```python
from build123d import *

# Parameters (mm, degrees)
BOSS_EXTRUDE1_DEPTH      = 1.5875
BOSS_EXTRUDE1_DEPTH_BACK = 1.5875
FILLET1_R                = 1.524
BOSS_EXTRUDE2_DEPTH      = 0.89581
BOSS_EXTRUDE2_DEPTH_BACK = 0.89581
FILLET2_R                = 1.016


with BuildPart() as part:
    # Sketch1 → Boss-Extrude1 (new, two sides: drawn at the far end of the back side and taken through both)
    with BuildSketch(Plane(origin=(0, 0, 0), x_dir=(1, 0, 0), z_dir=(0, 1, 0)).offset(-BOSS_EXTRUDE1_DEPTH_BACK)):
        with BuildLine():
            Line((-0.068296764, 6.214618695), (-0.068296764, 13.71487153))
            Line((-0.068296764, 13.71487153), (-0.895808533, 13.71487153))
            add(Edge.make_bspline(
                [(-0.895808533, 13.71487153), (-0.895808533, 4.54222596), (-1.588668774, 2.219313027), (-2.088196173, 1.337696034), (0, 0.766240154)],
                knots=[0, 0, 0, 0, 0, 1, 1, 1, 1, 1], degree=4))
            add(Edge.make_bspline(
                [(0.895808533, 13.71487153), (0.895808533, 4.54222596), (1.588668774, 2.219313027), (2.088196173, 1.337696034), (0, 0.766240154)],
                knots=[0, 0, 0, 0, 0, 1, 1, 1, 1, 1], degree=4))
            Line((0.895808533, 13.71487153), (0.068296764, 13.71487153))
            Line((0.068296764, 13.71487153), (0.068296764, 6.214618695))
            add(Edge.make_bspline(
                [(0.690807422, 2.606475487), (0.218071276, 3.482132924), (0.068296764, 6.214618695)],
                knots=[0, 0, 0, 1, 1, 1], degree=2))
            ThreePointArc((0.690807422, 2.606475487), (0, 1.52287153), (-0.690807422, 2.606475487))
            add(Edge.make_bspline(
                [(-0.690807422, 2.606475487), (-0.217222133, 3.738734236), (-0.068296764, 6.214618695)],
                knots=[0, 0, 0, 1, 1, 1], degree=2))
        make_face()
    extrude(amount=BOSS_EXTRUDE1_DEPTH + BOSS_EXTRUDE1_DEPTH_BACK)

    # Fillet1
    fillet1_edges = [part.edges().sort_by_distance(p)[0] for p in [
        (0, -0.79375, -0.766240154),
    ]]
    fillet(fillet1_edges, radius=FILLET1_R)

    # Sketch2 → Boss-Extrude2 (add, two sides: drawn at the far end of the back side and taken through both)
    with BuildSketch(Plane(origin=(0, 0, 0), x_dir=(0, 0, -1), z_dir=(1, 0, 0)).offset(-BOSS_EXTRUDE2_DEPTH_BACK)):
        Polygon((13.71487153, 1.5875), (13.71487153, -1.5875), (13.71487153, -23.8125), (14.73087153, -23.8125), (14.73087153, 1.5875), align=None)
    extrude(amount=BOSS_EXTRUDE2_DEPTH + BOSS_EXTRUDE2_DEPTH_BACK)

    # Fillet2
    fillet2_edges = [part.edges().sort_by_distance(p)[0] for p in [
        (0, 1.5875, -14.73087153),
        (0.482052648, -1.5875, -13.71487153),
        (-0.482052648, -1.5875, -13.71487153),
    ]]
    fillet(fillet2_edges, radius=FILLET2_R - 0.0001)  # a hair under: the kernel refuses the full size


solid = part.part
```
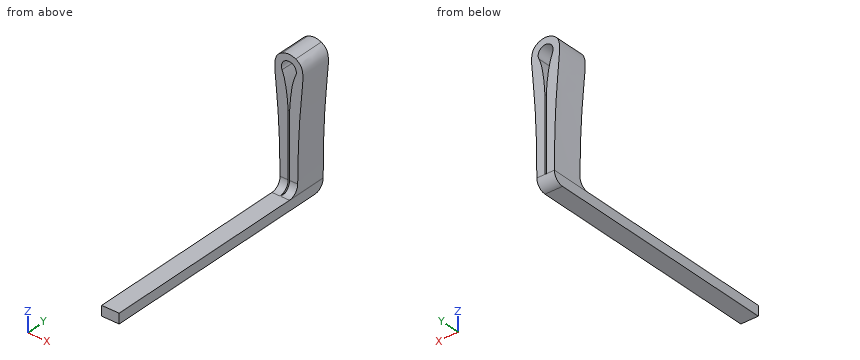
CAD build for the part. Positions are in the model's coordinates, mm. Round coordinates to 2 decimals unless told otherwise and drop trailing zeros. Order: outer loops, then holes, each group sorted by start corner. A loop starts at its lowest first (then second) coordinate and runs counter-clockwise, first axis right, second up. Notation, with made-up numbers: (-28.75, 73.5) -> (27.25, 73.5) arc R38 ccw to (27.25, 111.5) -> close; hole circle Ø5 at (42.25, 49). An arc over 180 degrees is marked (long way). Write item = value, one per line.
(1) Drill centre lines: L1, parallel to Z at x = 0, y = -0.3; L2, parallel to Y at x = -0.7, z = -3.5; L3, parallel to Z at x = -0.8, y = -7.5. Where is each one in solid material? Low to high.
Answers follow:
L1 = -14.73 to -13.71, -1.52 to -0.85
L2 = -1.59 to 1.59
L3 = -14.73 to -13.71
(2) Flat gauge pins, fed straight in: P1, Ø2, axis at y = -1, z = -9, coming from the +X side; P2, Ø3, axis at y = -9, z = -12, coming from the -X side; P3, Ø1.1, axis at y = -11.5, z = -14, coming from the -X side; P4, Ø1.4, axis at x = -0.5, z = -6.5, coming from the -Y side. Where does each tip first touch, or does it go through?
Answers follow:
P1 = 1.02
P2 = through
P3 = -0.9
P4 = -1.59
(3) Cut at A-A (y = -19.75). Write the cut outline in (x, z), plus the area to 3 significant figures.
Answers follow:
outline = (-0.9, -14.73) -> (0.9, -14.73) -> (0.9, -13.71) -> (-0.9, -13.71) -> close
area = 1.82 mm²
